Part print with two shaded views. Sizes in mm from the minimum x, y, z corner. A direction names the side the tool comes from. Give positions to 0.01 mm unless a question says otherwise; leave off trailing zeros. Order: outer loops, then holes, each group sorted by start corner. A loop starts at its lowest first (then second) coordinate and runs counter-clockwise, first axis right, second up. Notation, with made-up numbers: M 84,60 L 128,60 A7 cw 128,73 Z; hole C 75.25,28.5 d11. An arc over 180 degrees is marked long. Return JSON: item names as keys, results as strings.
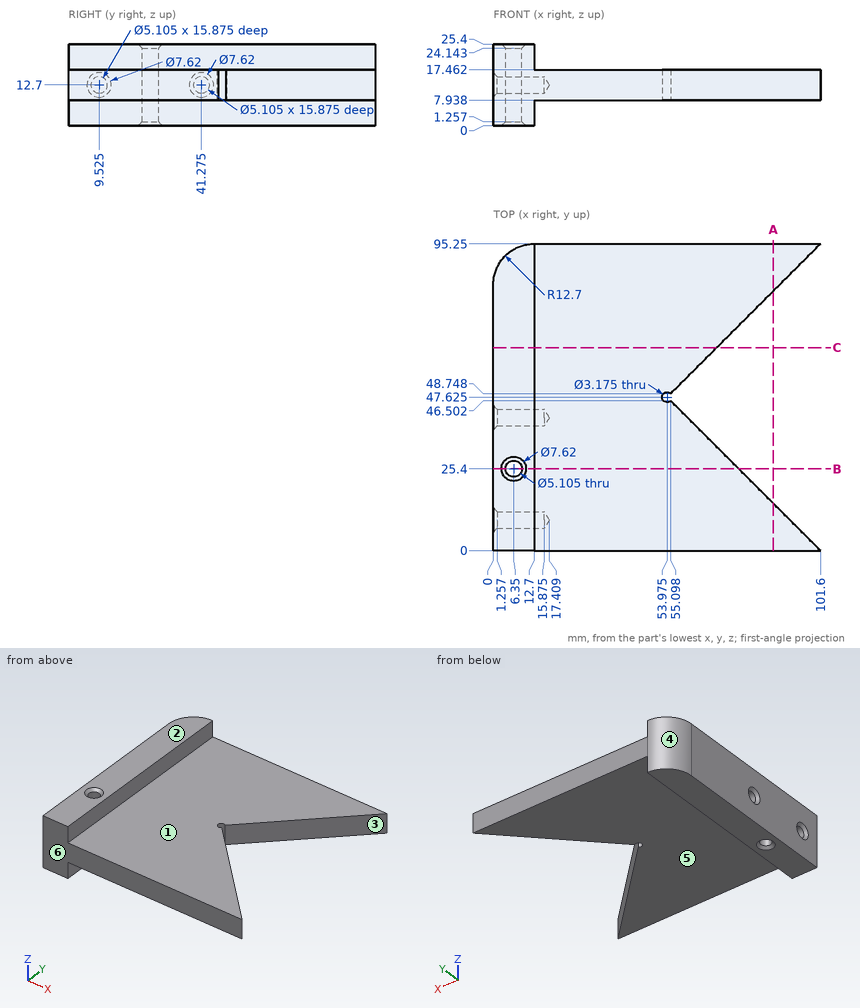
Q1. Band-saw the part on C-C (y = 63). Give the cut face in (x, z), then the cut area to 3 significant figures.
Established:
{"outline": "M 0,0 L 12.7,0 L 12.7,7.94 L 69.35,7.94 L 69.35,17.46 L 12.7,17.46 L 12.7,25.4 L 0,25.4 Z", "area": "862 mm²"}
Q2. Band-saw the part on A-A (x = 87). Give the cut face in (y, z).
Established:
{"outline": "M 0,7.94 L 14.6,7.94 L 14.6,17.46 L 0,17.46 Z; M 80.65,7.94 L 95.25,7.94 L 95.25,17.46 L 80.65,17.46 Z"}
Q3. Two-plate mould, pull along Y, no slides. Class the marked faces 3, 4, 5 and 6: +Y half, -Y half, draft (parallel to the pull), parting line (faces both ways), or undercut.
Established:
{"face 3": "undercut", "face 4": "+Y half", "face 5": "draft", "face 6": "-Y half"}
Q4. 3-axis set-ups, long thin cutter, end or side, ignore diameter. For the marked faces 1 and 2: which of +Z, -Z, +X, -X, +Y, -Y reach the whole face in a straight line?
Established:
{"face 1": "+Z, +X, +Y, -Y", "face 2": "+Z, +X, -X, +Y, -Y"}
Q5. Probe line 1 along Y through (x, z) = (10.5, 12.7); line 2 along X through (y, z) = (25.4, 7.75); line 3 along Y through (x, z) = (10, 12.7). List the from-to ranges inside material, lowest first.
Established:
{"line 1": "y = 0 to 6.97, 12.08 to 38.72, 43.83 to 95.06", "line 2": "x = 0 to 3.8, 8.9 to 12.7", "line 3": "y = 0 to 6.97, 12.08 to 38.72, 43.83 to 94.96"}
Q6. Pin check, flat tips, straight feed: pin 1 (6 mm diameter, centred on x = 74.5, y = 32, fed in from -Z); pin 2 (2 mm diameter, centred on x = 60, z = 14, fed in from -Y); pin 3 (2.5 mm diameter, centred on y = 68, z = 21, fed in from +X); pin 4 (4 mm diameter, centred on x = 53.975, y = 47.625, fed in from -Z). Stop position of each tip, or through.
Established:
{"pin 1": "passes through", "pin 2": "stops at y = 0", "pin 3": "stops at x = 12.7", "pin 4": "stops at z = 7.94"}
Q7. Band-saw the part on B-B (y = 25.4). Give the cut face in (x, z).
Established:
{"outline": "M 0,0 L 2.54,0 L 3.8,1.26 L 3.8,24.14 L 2.54,25.4 L 0,25.4 Z; M 8.9,1.26 L 10.16,0 L 12.7,0 L 12.7,7.94 L 76.2,7.94 L 76.2,17.46 L 12.7,17.46 L 12.7,25.4 L 10.16,25.4 L 8.9,24.14 Z"}
